Can you work these out from the model? Positions are in its coordinate system, mm. Face numbers are marked on the shaded views. A direction names the side the tool comes from. Coordinates: 2 decimals unless noted, no trailing zeros. Order: outer loops, then holes, each group sorted by start corner. A loop starts at its lowest first (then second) coordinate and runs counter-clockwise, first axis right, second up. Notation, with made-up numbers: (-30.75, 7.5) -> (-25.75, 7.5) arc R16 cw to (-25.75, 24.5) -> close; hole circle Ø4 at (-17.75, 38.5). An arc over 180 degrees is marked (long way). Use a Markdown table: item, result. Add a question column.
1. For pin 1 Ø17.5 at (x, z) = (8, 45.5) entering from -Y; pin 2 Ø11.5 at (x, z) = (0, 38.37) entering from +Y; pin 3 Ø1.5 at (x, y) = (18, -4) entering from -Z, each with a flat end and sliding along its axis, tell me the tip position at first contact or that it passes through.
2. If I drill on line 1 along Z through (x, y) = (0, 9.15); line 2 along X through (y, z) = (4, 110); line 3 along Z through (x, y) = (-14.5, 10.25), over which ranges is the centre line in solid material (lowest first)? Write a range as from..to.
3. Suppose I cut it at B-B, the plane x = 0. List the corners of the cut face in (y, z) for me, then the cut area to 3 significant figures.
4. Suppose I cut it at D-D, the plane z = 110. List the corners of the cut face in (x, y) for me.
5. Suppose I cut it at A-A, the plane z = 0. List the corners of the cut face in (x, y) for me, then the cut area to 3 significant figures.
6. Suppose I cut it at C-C, the plane y = 4. List the corners of the cut face in (x, z) for me, then the cut area to 3 significant figures.
7. For the marked faces 1, 2, 3, 4 and 5, which set-ups out of +Z, -Z, +X, -X, +Y, -Y let a thin tool reach every point of the face, with its end or its side?
8. We'd pull the mould along X, two halves only. Please class the marked faces 6, 7 and 8: pulls with the +X half, pulls with the -X half, needs draft (parallel to the pull), parting line crosses it, or undercut.
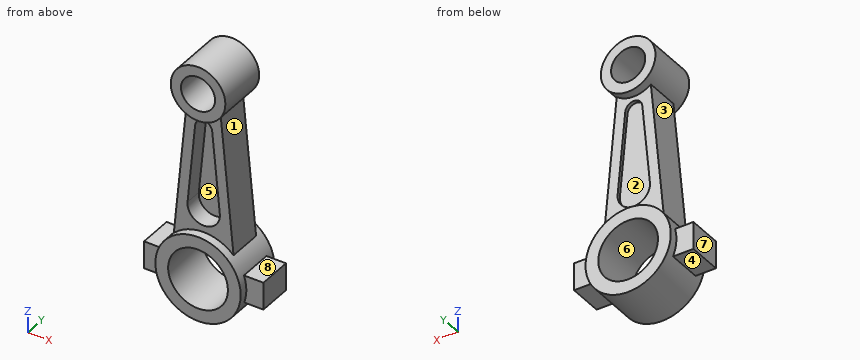
Autodesk Fusion 360 part; units mm, degrees
sketch "Sketch1" plane through (0, 0, 0) normal (0, 1, 0) x (1, 0, 0)
  circle A0 centre (0, 0) radius 17.5
  circle A1 centre (0, 0) radius 25
  circle A2 centre (0, -110) radius 10
  circle A3 centre (0, -110) radius 16
  line L0 (-10, -97.51) -> (-17.5, -17.8536)
  line L1 (10, -97.51) -> (17.5, -17.8536)
  line L2 (-23.0003, 9.7972) -> (-34.9353, 9.7972)
  line L3 (-34.9353, 9.7972) -> (-34.9353, -6.2028)
  line L4 (-14.9353, 9.7972) -> (-34.9353, -6.2028) construction
  line L5 (-34.9353, 9.7972) -> (-14.9353, -6.2028) construction
  line L6 (34.9986, -8.2633) -> (34.9986, 7.7367)
  line L7 (34.9986, 7.7367) -> (14.9986, -8.2633) construction
  line L8 (14.9986, 7.7367) -> (34.9986, -8.2633) construction
  line L9 (-34.9353, -6.2028) -> (-24.2183, -6.2028)
  line L10 (23.5949, -8.2633) -> (34.9986, -8.2633)
  line L11 (34.9986, 7.7367) -> (23.7727, 7.7367)
  arc A4 (9.4582, -39.2577) -> (-9.4582, -39.2577) centre (0, -38.3672) ccw
  arc A5 (-4.978, -86.8411) -> (4.978, -86.8411) centre (0, -86.3724) ccw
  line L12 (-4.978, -86.8411) -> (-9.4582, -39.2577)
  line L13 (4.978, -86.8411) -> (9.4582, -39.2577)
  point P0 (-24.9353, 1.7972)
  point P1 (24.9986, -0.2633)
  dimension "d1" = 35
  dimension "d2" = 50
  dimension "d3" = 20
  dimension "d4" = 32
  dimension "d5" = 110
  dimension "d6" = 20
  dimension "d7" = 35
  dimension "d10" = 5
  dimension "d11" = 9.5
  dimension "d12" = 16
  dimension "d13" = 20
  dimension "d14" = 16
  dimension "d15" = 20
extrude "Extrude1" add sketch "Sketch1" along normal mid plane 30 contours A1 | A3 makes body 1 at (17.413, 10, 1.7424) makes body 2 at (15.9205, 5, 108.4069)
extrude "Extrude2" add sketch "Sketch1" along normal mid plane 20 contours A1 L6 L10 L11 | A1 L2 L3 L9 | A1 A3 L0 L1 bodies 1 2
extrude "Extrude3" add sketch "Sketch1" along normal blind 8 contours A4 A5 L12 L13 bodies 1
Worked out:
| question | item | result |
|---|---|---|
| 1 | pin 1 | stops at y = -10 |
| 1 | pin 2 | stops at y = 8 |
| 1 | pin 3 | stops at z = -18.1 |
| 2 | line 1 | z = -25..-17.5, 17.5..28.87, 91.37..100, 120..126 |
| 2 | line 2 | x = -16..-10, 10..16 |
| 2 | line 3 | z = -20.37..-9.8, 9.8..20.37, 103.24..116.76 |
| 3 | outline | (-15, -25) -> (15, -25) -> (15, -17.5) -> (-15, -17.5) -> close; (-15, 17.5) -> (15, 17.5) -> (15, 25) -> (10, 25) -> (10, 28.87) -> (8, 28.87) -> (8, 91.37) -> (10, 91.37) -> (10, 94) -> (15, 94) -> (15, 100) -> (-15, 100) -> (-15, 94) -> (-10, 94) -> (-10, 91.37) -> (0, 91.37) -> (0, 28.87) -> (-10, 28.87) -> (-10, 25) -> (-15, 25) -> close; (-15, 120) -> (15, 120) -> (15, 126) -> (-15, 126) -> close |
| 3 | area | 1,440 mm² |
| 4 | outline | (-16, -15) -> (-10, -15) -> (-10, 15) -> (-16, 15) -> close; (10, -15) -> (16, -15) -> (16, 15) -> (10, 15) -> close |
| 5 | outline | (-34.94, -10) -> (-25, -10) -> (-25, -15) -> (-17.5, -15) -> (-17.5, 15) -> (-25, 15) -> (-25, 10) -> (-34.94, 10) -> close; (17.5, -15) -> (25, -15) -> (25, -10) -> (35, -10) -> (35, 10) -> (25, 10) -> (25, 15) -> (17.5, 15) -> close |
| 5 | area | 849 mm² |
| 6 | outline | (-34.94, -9.8) -> (-23, -9.8) arc R25 ccw to (23.77, -7.74) -> (35, -7.74) -> (35, 8.26) -> (23.59, 8.26) arc R25 ccw to (17.5, 17.85) -> (10, 97.51) arc R16 ccw (long way) to (-10, 97.51) -> (-17.5, 17.85) arc R25 ccw to (-24.22, 6.2) -> (-34.94, 6.2) -> close; hole circle Ø35 at (0, 0); hole circle Ø20 at (0, 110) |
| 6 | area | 3,800 mm² |
| 7 | face 1 | +X, +Y, -Y |
| 7 | face 2 | +Y |
| 7 | face 3 | -X, +Y, -Y |
| 7 | face 4 | -Z, -X, +Y, -Y |
| 7 | face 5 | -Y |
| 8 | face 6 | undercut |
| 8 | face 7 | pulls with the -X half |
| 8 | face 8 | needs draft |
